Check sheet for the modelled part. Datum: model origin and axes. Units: mm. A direction names the side the tool comes from. Round coordinates to 2 decimals unless told otherwise and drop trailing zeros. Order: outer loops, then holes, each group sorted by start corner. A loop starts at its lowest first (then second) coordinate and runs counter-clockwise, first axis right, second up.
Q1. Set-up check for faces 1 (the flat face through (5.82, 3.82, 2.54)), 2 (the flat face through (3, 0, 4)), 3 (the flat face through (1, 5, -1)): record each of +Z, -Z, +X, -X, +Y, -Y from which the full face is reachable in a straight line by a thin tool's end or side.
Q2. Scan lines: probe 1 along X at (y, z) = (5, 4.3) (3 decimals); probe 2 along Y at (x, z) = (4.7, 4.25) (3 decimals); probe 3 along Z at (x, y) = (1.5, 1.5). Record each from-to range of solid material in increasing order.
Q3. Depth check by flat-ended pin: P1, Ø0.6, axis at y = 5, z = -0.5, coming from the +X side. Enter the tip coordinate at first touch or a pass-through.
Q4. Cross-section at C-C on y = 9.25. Record the cut outline in (x, z).
Q5. Cross-section at B-B on x = 5.25. Record the cut outline in (y, z).
Q6. Cross-section at D-D on z = -1.5. Record the cut outline in (x, y), then the cut area to 3 significant figures.
Q7. Cross-section at A-A on y = 4.75. Record the cut outline in (x, z), then the cut area to 3 significant figures.
from build123d import *

# Parameters (mm, degrees)
SKETCH2_W           = 1.2
SKETCH2_H           = 10
SKETCH2_W_2         = 1
BOSS_EXTRUDE1_DEPTH = 5
SKETCH2_3_W         = 1
SKETCH2_3_H         = 10
BOSS_EXTRUDE2_DEPTH = 2
BOSS_EXTRUDE3_DEPTH = 6
SKETCH4_R           = 1.125
CUT_EXTRUDE1_DEPTH  = 6


with BuildPart() as part:
    # Sketch2 → Boss-Extrude1 (new body)
    with BuildSketch(Plane.XY):
        with Locations((1.6, 5)):
            Rectangle(SKETCH2_W, SKETCH2_H)
        with Locations((0.5, 5)):
            Rectangle(SKETCH2_W_2, SKETCH2_H)
    extrude(amount=BOSS_EXTRUDE1_DEPTH)

    # Sketch2_3 → Boss-Extrude2 (add)
    with BuildSketch(Plane.XY):
        with Locations((0.5, 5)):
            Rectangle(SKETCH2_3_W, SKETCH2_3_H)
    extrude(amount=-BOSS_EXTRUDE2_DEPTH)

    # Sketch3 → Boss-Extrude3 (add)
    with BuildSketch(Plane(origin=(2.2, 0, 0), x_dir=(0, 0, -1), z_dir=(1, 0, 0))):
        Polygon((-5, 0), (-3.52903009, 0), (-0.942854246, 10), (-5, 10), align=None)
    extrude(amount=BOSS_EXTRUDE3_DEPTH)

    # Sketch4 → Cut-Extrude1 (cut)
    with BuildSketch(Plane.XY.offset(5)):
        with Locations((4.7, 5)):
            Circle(SKETCH4_R)
    extrude(amount=-CUT_EXTRUDE1_DEPTH, mode=Mode.SUBTRACT)


solid = part.part
Results found:
1. face 1: -Z, +X, -Y
1. face 2: +Z, -Z, +X, -X, -Y
1. face 3: -Z, +X, +Y, -Y
2. probe 1: x = 0 to 3.575, 5.825 to 8.2
2. probe 2: y = 0 to 3.875, 6.125 to 10
2. probe 3: z = 0 to 5
3. P1: stops at x = 1
4. outline: (0, -2) - (1, -2) - (1, 0) - (2.2, 0) - (2.2, 1.14) - (8.2, 1.14) - (8.2, 5) - (0, 5) - close
5. outline: (0, 3.53) - (4.02, 2.49) - (4.02, 5) - (0, 5) - close; (5.98, 1.98) - (10, 0.94) - (10, 5) - (5.98, 5) - close
6. outline: (0, 0) - (1, 0) - (1, 10) - (0, 10) - close
6. area: 10.0 mm2
7. outline: (0, -2) - (1, -2) - (1, 0) - (2.2, 0) - (2.2, 2.3) - (3.6, 2.3) - (3.6, 5) - (0, 5) - close; (5.8, 2.3) - (8.2, 2.3) - (8.2, 5) - (5.8, 5) - close
7. area: 23.3 mm2
